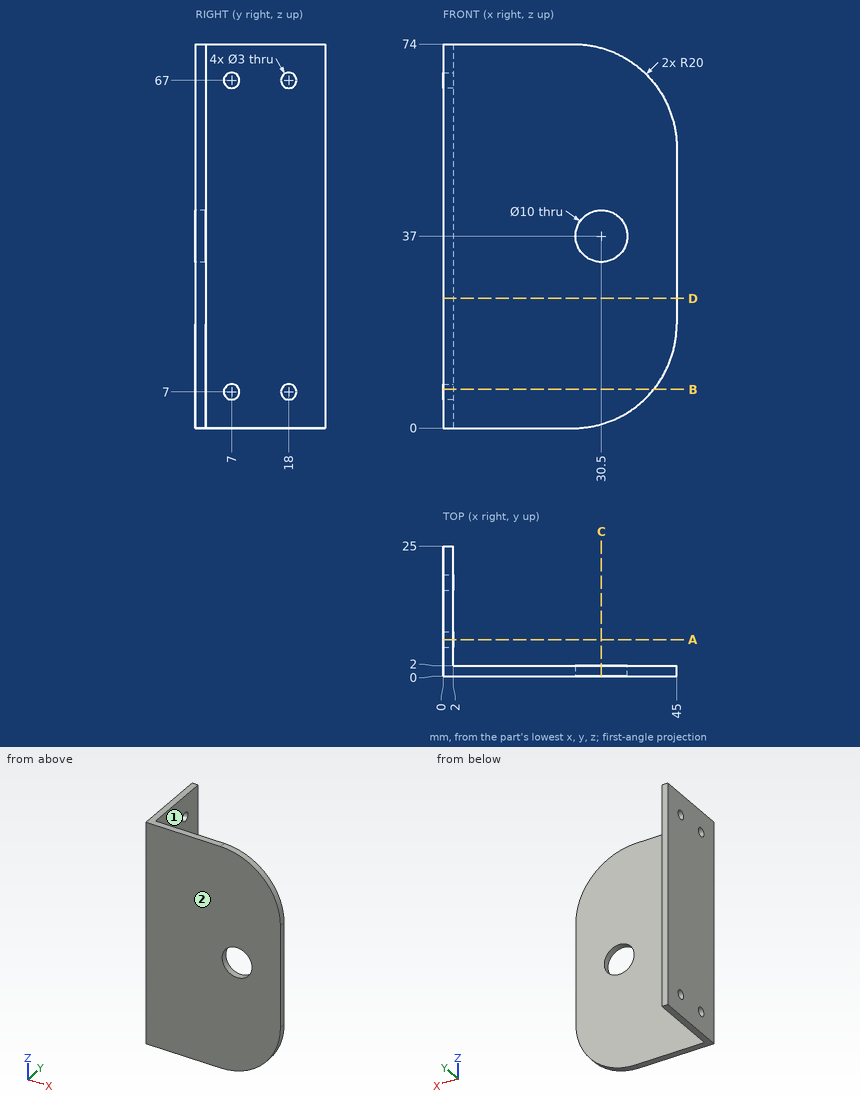
Geometry: see drawing. Coordinates: mm, zero at the bounding-box minimum. A direction names the side the tool comes from. Coordinates: 2 decimals unless noted, no trailing zeros. Order: outer loops, then holes, each group sorted by start corner. A loop starts at its lowest first (then second) coordinate and runs counter-clockwise, first axis right, second up. Notation, with made-up numbers: (42.5, 30) -> (71.5, 30) arc R16 ccw to (71.5, 42) -> close; hole circle Ø8 at (86, -2). An arc over 180 degrees is marked (long way). Write each question's results on one line, items separated by ' | '. Start each with the question number.
1) Cut plane B-B, the plane z = 7.5. Output: boundary loops of the cut face in (x, y), and give its area (3 significant figures).
2) Cut plane C-C, the plane x = 30.5. Output: boundary loops of the cut face in (y, z).
3) Cut plane D-D, the plane z = 25. Output: boundary loops of the cut face in (x, y), and give its area (3 significant figures).
4) Material intervals for line 1 along Y through (x, z) = (1.2, 7); line 2 along X through (y, z) = (13, 67.5), sorted ascending.
5) First-contact query: pin 1 (4 mm diameter, centred on x = 35, z = 10, fed in from -Y); pin 2 (3 mm diameter, centred on x = 16, z = 37.5, fed in from +Y); pin 3 (6 mm diameter, centred on y = 22, z = 49.5, fed in from +X). Flat tips, straight axial feed; report the tip coordinate or a pass-through.
6) Set-up query: the marked faces 1 and 2. Return all of +Z, -Z, +X, -X, +Y, -Y with unobstructed straight access to the full face (end or side cutting, diameter ignored); none if empty.
7) Cut plane A-A, the plane y = 7. Output: boundary loops of the cut face in (x, z), and give its area (3 significant figures).
Checks:
1) outline: (0, 0) -> (40.61, 0) -> (40.61, 2) -> (2, 2) -> (2, 5.59) -> (0, 5.59) -> close; (0, 8.41) -> (2, 8.41) -> (2, 16.59) -> (0, 16.59) -> close; (0, 19.41) -> (2, 19.41) -> (2, 25) -> (0, 25) -> close | area: 116 mm^2
2) outline: (0, 0.77) -> (2, 0.77) -> (2, 32) -> (0, 32) -> close; (0, 42) -> (2, 42) -> (2, 73.23) -> (0, 73.23) -> close
3) outline: (0, 0) -> (45, 0) -> (45, 2) -> (2, 2) -> (2, 25) -> (0, 25) -> close | area: 136 mm^2
4) line 1: 0 to 5.5, 8.5 to 16.5, 19.5 to 25 | line 2: 0 to 2
5) pin 1: y = 0 | pin 2: y = 2 | pin 3: x = 2
6) face 1: +Z, -Z, +X, +Y | face 2: +Z, -Z, +X, -X, -Y
7) outline: (0, 0) -> (2, 0) -> (2, 5.5) -> (0, 5.5) -> close; (0, 8.5) -> (2, 8.5) -> (2, 65.5) -> (0, 65.5) -> close; (0, 68.5) -> (2, 68.5) -> (2, 74) -> (0, 74) -> close | area: 136 mm^2
